Design review of the part shown in the three views and the two pictorial views. Dimensions are in mm from the part's minimum x, y and z. A direction names the side the tool comes from. Coordinates: 2 decimals unless noted, no trailing zeros. Loops run counter-clockwise (first coordinate to the right, second up) from the corner with the lowest first, then second, coordinate; pieces in that order, holes last. Notation, with made-up numbers: (36.25, -2) -> (70.25, -2) arc R30 cw to (70.25, 27) -> close; hole circle Ø10 at (86, 77.5). An arc over 180 degrees is marked (long way). One line per item, written item: value.
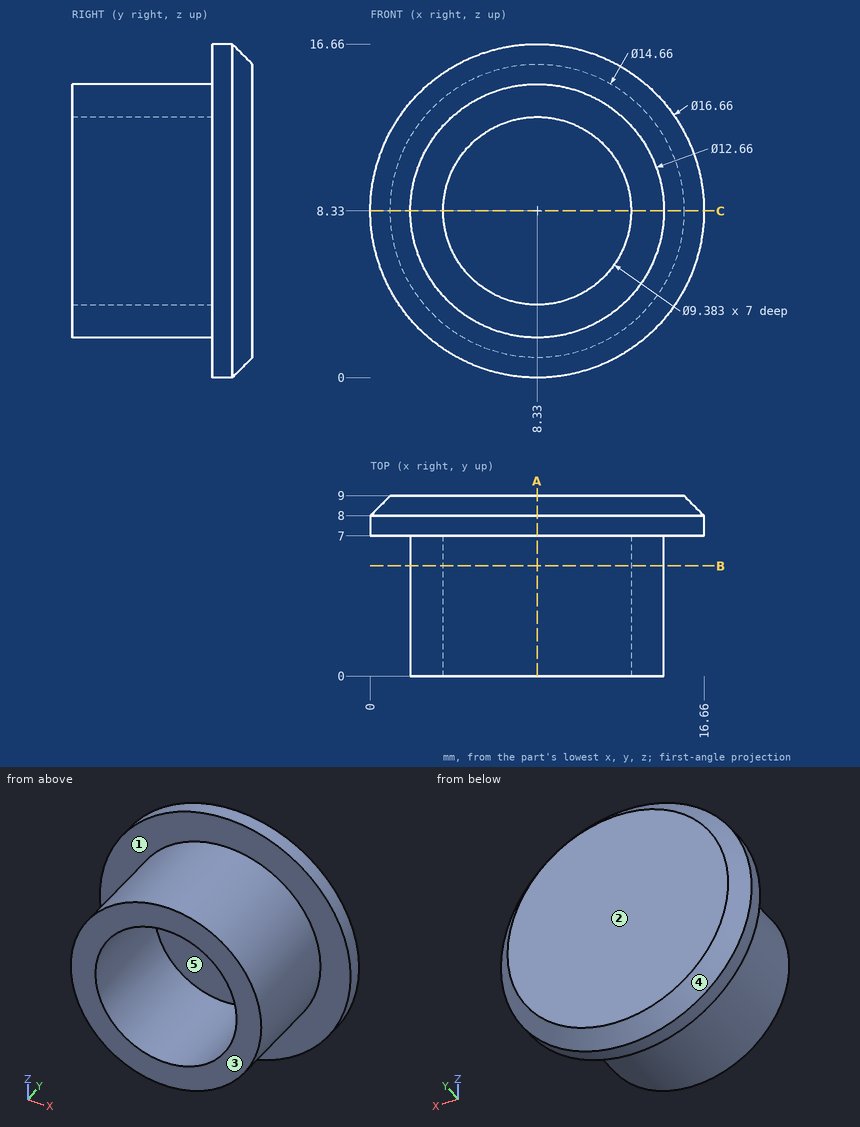
1. To check wall thickness, follow probe 1 along X at (y, z) = (2.25, 8.33); probe 2 along Y at (x, z) = (7.5, 1.25). State the ranges of each line that lie inside material, in increasing order. Write a range as from..to.
Return value:
probe 1: x = 2..3.64, 13.02..14.66
probe 2: y = 7..9
2. Take a section at B-B, the plane y = 5.5. Give the boundary of the cut face in (x, z).
Return value:
outline: circle Ø12.66 at (8.33, 8.33); hole circle Ø9.38 at (8.33, 8.33)
3. Insertion check: pin 1 Ø1 at (x, z) = (6.5, 8) entering from -Y; pin 2 Ø4 at (y, z) = (5.5, 2.5) entering from -X (1 decimal); pin 3 Ø1 at (y, z) = (2.5, 8) entering from -X. Each pin has a flat end and moves straight along its axis. Give the tip position at first contact, or say it passes through.
Return value:
pin 1: stops at y = 7
pin 2: stops at x = 1.3
pin 3: stops at x = 2
4. The part is to be moulded in two halves that separate along Z. For the marked faces 3, 4 and 5, say which applies: pulls with the +Z half, pulls with the -Z half, needs draft (parallel to the pull), parting line crosses it, or undercut.
Return value:
face 3: needs draft
face 4: parting line crosses it
face 5: undercut
5. Take a section at A-A, the plane x = 8.33. Give the boundary of the cut face in (y, z).
Return value:
outline: (0, 2) -> (7, 2) -> (7, 0) -> (8, 0) -> (9, 1) -> (9, 15.66) -> (8, 16.66) -> (7, 16.66) -> (7, 14.66) -> (0, 14.66) -> (0, 13.02) -> (7, 13.02) -> (7, 3.64) -> (0, 3.64) -> close
6. Take a section at C-C, the plane z = 8.33. Give the boundary of the cut face in (x, y).
Return value:
outline: (0, 7) -> (2, 7) -> (2, 0) -> (3.64, 0) -> (3.64, 7) -> (13.02, 7) -> (13.02, 0) -> (14.66, 0) -> (14.66, 7) -> (16.66, 7) -> (16.66, 8) -> (15.66, 9) -> (1, 9) -> (0, 8) -> close
7. For the marked faces 1 and 2, list the 3-axis set-ups (+Z, -Z, +X, -X, +Y, -Y) from which the entire face can be reached by the end or side of a thin tool; tool diameter is ignored.
Return value:
face 1: -Y
face 2: +Z, -Z, +X, -X, +Y
